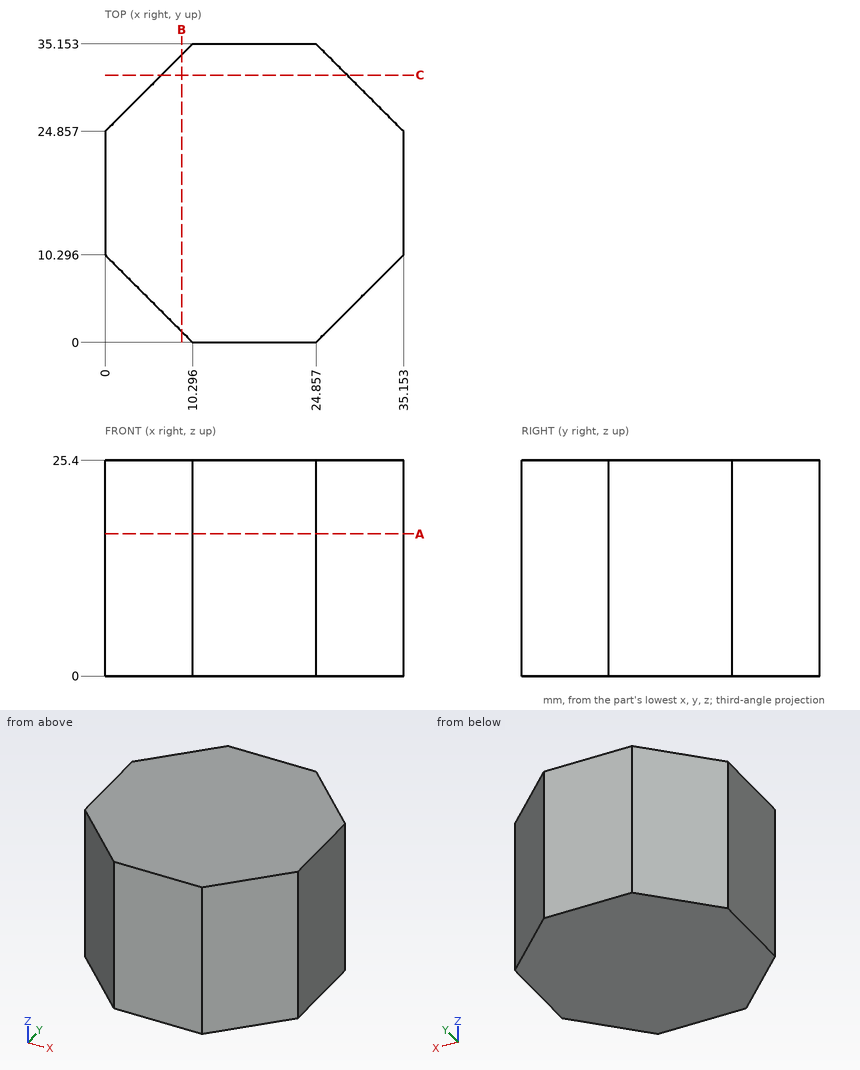
Here's the drawing with two shaded views (mm, measured from the low corner). I have some questions. Give positions to 0.01 mm unless a question says otherwise; leave off trailing zeros. Order: outer loops, then holes, each group sorted by start corner. A loop starts at its lowest first (then second) coordinate and runs counter-clockwise, first axis right, second up. Notation, with made-up numbers: (41, 60.5) -> (50, 60.5) arc R27 cw to (50, 83.5) -> close; hole circle Ø4 at (38, -21). An arc over 180 degrees is marked (long way). Use a Markdown table: item, result. Add a question column.
Item 1: Imagine slicing it at C-C on y = 31.5. Please give me the cut outline in (x, z), plus the area to 3 significant figures.
Item 2: Will these pins go through, and if not, where does the flat tip stop? pin 1 (1.5 mm diameter, centred on x = 31.5, z = 6.5, fed in from -Y); pin 2 (1.5 mm diameter, centred on y = 9.5, z = 16.5, fed in from -X) (1 decimal).
Item 3: I need wall thicknesses on line 1 (X direction, y = 6.5, z = 4) (1 decimal); line 2 (X direction, y = 34, z = 13) (1 decimal); line 3 (Y direction, x = 32.5, z = 10.5) (1 decimal). Which ranges of each line are inside material? Lowest first, please.
Item 4: Imagine slicing it at A-A on z = 16.75. Please give me the cut outline in (x, y).
Item 5: Imagine slicing it at B-B on x = 9. Please give me the cut outline in (y, z), plus the area to 3 significant figures.
Data:
| question | item | result |
|---|---|---|
| 1 | outline | (6.64, 0) -> (28.51, 0) -> (28.51, 25.4) -> (6.64, 25.4) -> close |
| 1 | area | 555 mm² |
| 2 | pin 1 | stops at y = 5.89 |
| 2 | pin 2 | stops at x = 0 |
| 3 | line 1 | x = 3.8 to 31.4 |
| 3 | line 2 | x = 9.1 to 26 |
| 3 | line 3 | y = 7.6 to 27.5 |
| 4 | outline | (0, 10.3) -> (10.3, 0) -> (24.86, 0) -> (35.15, 10.3) -> (35.15, 24.86) -> (24.86, 35.15) -> (10.3, 35.15) -> (0, 24.86) -> close |
| 5 | outline | (1.3, 0) -> (33.86, 0) -> (33.86, 25.4) -> (1.3, 25.4) -> close |
| 5 | area | 827 mm² |
